```python
from build123d import *

# Parameters (mm, degrees)
F1_DEPTH = 200
F2_T     = -1.2
F3_W     = 10
F3_H     = 2
F4_DEPTH = 1.2


with BuildPart() as f1:
    # F0 (on Top) → F1 (new body)
    with BuildSketch(Plane.XY):
        with BuildLine():
            Line((80, 100), (-90, 100))
            ThreePointArc((-90, 100), (-93.826834, 99.238795), (-97.071068, 97.071068))
            Line((-97.071068, 97.071068), (0, 0))
            Line((0, 0), (94.142136, 94.142136))
            ThreePointArc((94.142136, 94.142136), (87.653669, 98.477591), (80, 100))
        make_face()
        with BuildLine():
            ThreePointArc((100, 80), (98.477591, 87.653669), (94.142136, 94.142136))
            Line((94.142136, 94.142136), (0, 0))
            Line((0, 0), (97.071068, -97.071068))
            ThreePointArc((97.071068, -97.071068), (99.238795, -93.826834), (100, -90))
            Line((100, -90), (100, 80))
        make_face()
        with BuildLine():
            Line((97.071068, -97.071068), (0, 0))
            Line((0, 0), (-94.142136, -94.142136))
            ThreePointArc((-94.142136, -94.142136), (-87.653669, -98.477591), (-80, -100))
            Line((-80, -100), (90, -100))
            ThreePointArc((90, -100), (93.826834, -99.238795), (97.071068, -97.071068))
        make_face()
        with BuildLine():
            Line((0, 0), (-97.071068, 97.071068))
            ThreePointArc((-97.071068, 97.071068), (-99.238795, 93.826834), (-100, 90))
            Line((-100, 90), (-100, -80))
            ThreePointArc((-100, -80), (-98.477591, -87.653669), (-94.142136, -94.142136))
            Line((-94.142136, -94.142136), (0, 0))
        make_face()
    extrude(amount=F1_DEPTH)

    # F2
    f2_openings = [f1.faces().sort_by_distance(p)[0] for p in [
        (0, 0, 200),
    ]]
    offset(amount=F2_T, openings=f2_openings)


with BuildPart() as f4:
    # F3 (on face) → F4 (new body, through all)
    with BuildSketch(Plane(origin=(-100, 0, 0), x_dir=(0, -1, 0), z_dir=(-1, 0, 0))):
        with Locations((-45, 196)):
            Rectangle(F3_W, F3_H)
        with Locations((45, 196)):
            Rectangle(F3_W, F3_H)
    extrude(amount=-F4_DEPTH)


with BuildPart() as f5_1:
    # F5: instance of F4
    add(f4.part.mirror(Plane.YZ))


with BuildPart() as f1_1:
    add(f1.part)

    # F6: cut F4, F5_1
    add(f4.part, mode=Mode.SUBTRACT)
    add(f5_1.part, mode=Mode.SUBTRACT)


solid = f1_1.part
```
Read the model definition and answer for the solid it produces. Units are mm, in the model's axes. A direction names the side the tool comes from. Round coordinates to 2 decimals unless told otherwise and drop trailing zeros. Loops run counter-clockwise (first coordinate to the right, second up) from the corner with the lowest first, then second, coordinate; pieces in that order, holes last. Notation, with made-up numbers: (87.25, 27) -> (125.25, 27) arc R16 cw to (125.25, 41) -> close; hole circle Ø8 at (-26, 40.25). An arc over 180 degrees is marked (long way). One line per item, written item: value.
1) Flat-ended cylindrical pins translate along their axes: P1, Ø5, axis at x = 74.5, y = -73, coming from the +Z side; P2, Ø0.6, axis at x = 99.5, z = 196, coming from the -Y side; P3, Ø1, axis at x = 99.5, z = 195.5, coming from the -Y side. Find the tip coordinate at first contact, or state that the pin passes through.
Answer list:
P1: stops at z = 1.2
P2: stops at y = -93.92
P3: stops at y = -94.36
2) Consider L1, parallel to Y at x = 0, z = 137; L2, parallel to Z at x = -80.5, y = -16. Determine where each line is inside the solid, lowest interval first. Write a range as [from, to].
Answer list:
L1: y = [-100, -98.8], [98.8, 100]
L2: z = [0, 1.2]
3) For faces 1 (the face through (-1, 1, 1.2)), 2 (the face through (100, -6, 99)), determine the directions among +Z, -Z, +X, -X, +Y, -Y from which every point of the face is accessible in a straight line to the end or side of a thin tool.
Answer list:
face 1: +Z
face 2: +Z, -Z, +X, +Y, -Y
4) A cutting plane is placed at A-A (x = -6). Determine the outline of the cut face in (y, z), and give its area (3 significant figures).
Answer list:
outline: (-100, 0) -> (100, 0) -> (100, 200) -> (98.8, 200) -> (98.8, 1.2) -> (-98.8, 1.2) -> (-98.8, 200) -> (-100, 200) -> close
area: 717 mm²
5) A cutting plane is placed at B-B (z = 96.5). Determine the outline of the cut face in (x, y).
Answer list:
outline: (-100, -80) arc R20 ccw to (-80, -100) -> (90, -100) arc R10 ccw to (97.07, -97.07) arc R10 ccw to (100, -90) -> (100, 80) arc R20 ccw to (80, 100) -> (-90, 100) arc R10 ccw to (-97.07, 97.07) arc R10 ccw to (-100, 90) -> close; hole (-98.8, -80) arc R18.8 ccw to (-80, -98.8) -> (90, -98.8) arc R8.8 ccw to (96.22, -96.22) arc R8.8 ccw to (98.8, -90) -> (98.8, 80) arc R18.8 ccw to (80, 98.8) -> (-90, 98.8) arc R8.8 ccw to (-96.22, 96.22) arc R8.8 ccw to (-98.8, 90) -> close
